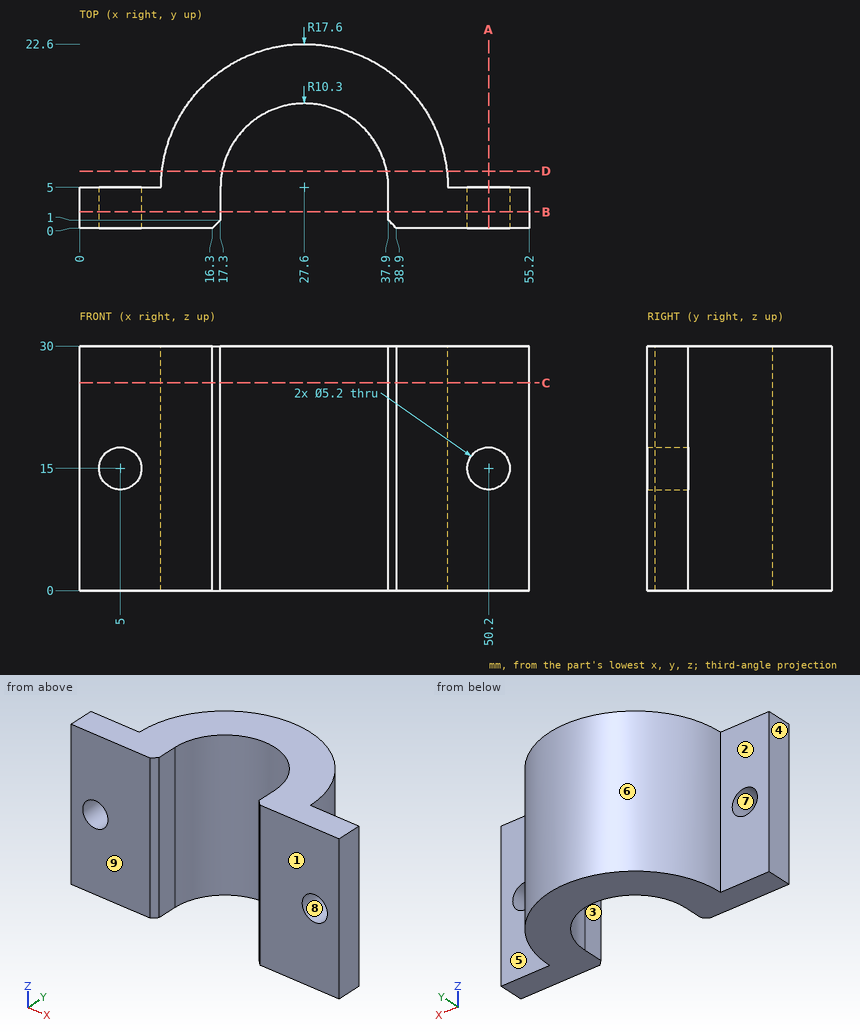
Can you work these out from the drawing? Everything is in mm from the part's minimum corner. A direction names the side the tool comes from. Give positions to 0.01 mm unless a question says otherwise; leave off trailing zeros. Order: outer loops, then holes, each group sorted by start corner. A loop starts at its lowest first (then second) coordinate and runs counter-clockwise, first axis right, second up. Notation, with made-up numbers: (-36.75, 73.5) -> (-2.75, 73.5) arc R16 ccw to (-2.75, 98.5) -> close; hole circle Ø11 at (5, -30.5). An arc over 180 degrees is marked (long way). Return JSON: item names as keys, results as strings.
1. Imagine slicing it at D-D on y = 7. List the corners of the cut face in (x, z) for me.
Answer list:
{"outline": "(10.11, 0) -> (17.5, 0) -> (17.5, 30) -> (10.11, 30) -> close; (37.7, 0) -> (45.09, 0) -> (45.09, 30) -> (37.7, 30) -> close"}
2. Imagine slicing it at A-A on x = 50.2. List the corners of the cut face in (y, z) for me.
Answer list:
{"outline": "(0, 0) -> (5, 0) -> (5, 12.4) -> (0, 12.4) -> close; (0, 17.6) -> (5, 17.6) -> (5, 30) -> (0, 30) -> close"}
3. On a 3-axis mill with a long thin cutter (end or side, diameter ignored), from which of +Z, -Z, +X, -X, +Y, -Y can I reach the whole of each face in a straight line? I mean the marked faces 1, 2, 3, 4 and 5. Say none if no direction works.
Answer list:
{"face 1": "+Z, -Z, +X, -X, -Y", "face 2": "+Z, -Z, -X, +Y", "face 3": "+Z, -Z, -Y", "face 4": "+Z, -Z, -X, +Y, -Y", "face 5": "+Z, -Z, +X, +Y"}
4. Imagine slicing it at C-C on z = 25.5. List the corners of the cut face in (x, y) for me.
Answer list:
{"outline": "(0, 0) -> (16.3, 0) -> (17.3, 1) -> (17.3, 5) arc R10.3 cw to (37.9, 5) -> (37.9, 1) -> (38.9, 0) -> (55.2, 0) -> (55.2, 5) -> (45.2, 5) arc R17.6 ccw to (10, 5) -> (0, 5) -> close"}
5. Imagine slicing it at B-B on y = 2. List the corners of the cut face in (x, z) for me, then the cut area to 3 significant figures.
Answer list:
{"outline": "(0, 0) -> (17.3, 0) -> (17.3, 30) -> (0, 30) -> close; (37.9, 0) -> (55.2, 0) -> (55.2, 30) -> (37.9, 30) -> close; hole circle Ø5.2 at (5, 15); hole circle Ø5.2 at (50.2, 15)", "area": "996 mm2"}
6. For pin 1 Ø1 at (x, z) = (6.5, 11) entering from +Y; pin 2 Ø1.5 at (x, z) = (21, 9) entering from +Y; pin 3 Ø4 at (x, z) = (22.5, 6.5) entering from +Y, each with a flat end and sliding along its axis, tell me the tip position at first contact or that it passes through.
Answer list:
{"pin 1": "stops at y = 5", "pin 2": "stops at y = 21.6", "pin 3": "stops at y = 22.32"}
7. I need wall thicknesses on line 1 (X direction, y = 3.4, z = 15); line 2 (X direction, y = 5.5, z = 18); line 3 (Z direction, x = 50.2, y = 3.7). Which ranges of each line are inside material? Lowest first, please. Write a range as from..to.
Answer list:
{"line 1": "x = 0..2.4, 7.6..17.3, 37.9..47.6, 52.8..55.2", "line 2": "x = 10.01..17.31, 37.89..45.19", "line 3": "z = 0..12.4, 17.6..30"}
8. Thinking about a two-plate mould opening in X: for the marked faces 6, 7, 8 and 9, which applies, pulls with the +X half, pulls with the -X half, needs draft (parallel to the pull), parting line crosses it, or undercut?
Answer list:
{"face 6": "parting line crosses it", "face 7": "undercut", "face 8": "undercut", "face 9": "needs draft"}
